from build123d import *

# Parameters (mm, degrees)
F0_W     = 10.2165445685
F0_H     = 50
F1_DEPTH = 25
F0_W_2   = 79.5669108629
F2_DEPTH = 10
F3_DEPTH = 25
F4_R     = 5
F5_R     = 5
F6_SIZE  = 5


with BuildPart() as f1:
    # F0 (on Top) → F1 (new body)
    with BuildSketch(Plane.XY):
        with Locations((-44.8917277157, 0)):
            Rectangle(F0_W, F0_H)
    extrude(amount=F1_DEPTH)

    # F0 (on Top) → F2 (join)
    with BuildSketch(Plane.XY):
        Rectangle(F0_W_2, F0_H)
    extrude(amount=F2_DEPTH)

    # F0 (on Top) → F3 (join)
    with BuildSketch(Plane.XY):
        with Locations((44.8917277157, 0)):
            Rectangle(F0_W, F0_H)
    extrude(amount=F3_DEPTH)

    # F4
    f4_edges = [f1.edges().sort_by_distance(p)[0] for p in [
        (50, 0, 25),
    ]]
    fillet(f4_edges, radius=F4_R)

    # F5
    f5_edges = [f1.edges().sort_by_distance(p)[0] for p in [
        (-50, 0, 25),
    ]]
    fillet(f5_edges, radius=F5_R)

    # F6
    f6_edges = [f1.edges().sort_by_distance(p)[0] for p in [
        (0, -25, 10),
    ]]
    chamfer(f6_edges, length=F6_SIZE)


solid = f1.part
Check sheet for the modelled part. Datum: model origin and axes. Units: mm. A direction names the side the tool comes from. Round coordinates to 2 decimals unless told otherwise and drop trailing zeros. Order: outer loops, then holes, each group sorted by start corner. A loop starts at its lowest first (then second) coordinate and runs counter-clockwise, first axis right, second up.
(1) Draft check along X on faces 1 (the flat face through (-50, 0, 10)), 2 (the flat face through (50, 0, 10)), 3 (the flat face through (-1, -22, 8)). Enter one of: pulls with the +X half, pulls with the -X half, needs draft (parallel to the pull), parting line crosses it, or undercut.
(2) Scan lines: probe 1 along X at (y, z) = (-21, 15.75); probe 2 along Z at (x, y) = (-25.5, 10.5); probe 3 along X at (y, z) = (3.5, 22.75). Record each from-to range of solid material in increasing order.
(3) Cross-section at C-C, the plane y = 13. Enter the section's corners in (x, z), and give its area (3 significant figures).
(4) Access from +Z, -Z, +X, -X, +Y, -Y to the whole of each face (thin tool, end or side, straight path). Record for faces 4 (the flat face through (-1, 3, 10)), 5 (the flat face through (-42, 0, 25)).
(5) Cross-section at B-B, the plane z = 6.5. Enter the section's corners in (x, y).
(6) Cross-section at A-A, the plane z = 17. Enter the section's corners in (x, y), and give its area (3 significant figures).
(7) Cross-section at D-D, the plane x = -30. Enter the section's corners in (y, z).
(8) Go/stop test with flat-tipped pins: P1, Ø8, axis at x = 30.5, y = 13.5, coming from the -Z side; P2, Ø12, axis at x = -3, z = 12, coming from the -Y side; P3, Ø22.5, axis at x = 0.5, y = -1.5, coming from the +Z side. Record where each tip stops, or that it passes through.
Check sheet entries:
1. face 1: pulls with the -X half
1. face 2: pulls with the +X half
1. face 3: undercut
2. probe 1: x = -50 to -39.78, 39.78 to 50
2. probe 2: z = 0 to 10
2. probe 3: x = -49.18 to -39.78, 39.78 to 49.18
3. outline: (-50, 0) - (50, 0) - (50, 20) arc R5 ccw to (45, 25) - (39.78, 25) - (39.78, 10) - (-39.78, 10) - (-39.78, 25) - (-45, 25) arc R5 ccw to (-50, 20) - close
3. area: 1,300 mm2
4. face 4: +Z, +Y, -Y
4. face 5: +Z, +X, -X, +Y, -Y
5. outline: (-50, -25) - (-39.78, -25) - (-39.78, -23.5) - (39.78, -23.5) - (39.78, -25) - (50, -25) - (50, 25) - (-50, 25) - close
6. outline: (-50, -25) - (-39.78, -25) - (-39.78, 25) - (-50, 25) - close; (39.78, -25) - (50, -25) - (50, 25) - (39.78, 25) - close
6. area: 1,020 mm2
7. outline: (-25, 0) - (25, 0) - (25, 10) - (-20, 10) - (-25, 5) - close
8. P1: stops at z = 0
8. P2: stops at y = -24
8. P3: stops at z = 10
